Can you work these out from the model? Positions are in its coordinate system, mm. Give positions to 0.01 mm unless a question says otherwise; leave off trailing zeros. Order: outer loops, then holes, each group sorted by start corner. A loop starts at its lowest first (then second) coordinate and runs counter-clockwise, first axis right, second up.
Item 1: I want a section at D-D, the plane z = 2.1. Write out the boundary of the cut face in (x, y) (3 decimals).
Item 2: I want a section at C-C, the plane x = 40. Write out the boundary of the cut face in (y, z) (3 decimals).
Item 3: If we mould it in two halves opening along Y, with no side actions, what happens to faces 1 (the flat face through (25, 0, 2)), 2 (the flat face through (25, -47, 5)), 3 (the cylindrical face through (24.57, -85.48, 2.46))? For each: +Y half, -Y half, draft (parallel to the pull), parting line (faces both ways), or undercut.
Item 4: I want a section at A-A, the plane x = 25. Write out the boundary of the cut face in (y, z) (3 decimals), then the cut area to 3 significant figures.
Item 5: I want a section at B-B, the plane y = -9.5. Write out the boundary of the cut face in (x, z).
Item 6: If I drill on line 1 along Y through (x, z) = (10, 1.25) (3 decimals); line 2 along Y through (x, z) = (25, 3.5) (3 decimals); line 3 along Y through (x, z) = (39, 0.9), over which ranges is the centre line in solid material (lowest first)?
```python
from build123d import *

# Parameters (mm, degrees)
SKETCH1_W           = 50
SKETCH1_H           = 95
SKETCH1_R           = 2.5
SKETCH1_R_2         = 8
SKETCH1_R_3         = 2
BOSS_EXTRUDE1_DEPTH = 5
FILLET1_R           = 5


with BuildPart() as part:
    # Sketch1 → Boss-Extrude1 (new body)
    with BuildSketch(Plane.XY):
        with Locations((25, -47.5)):
            Rectangle(SKETCH1_W, SKETCH1_H)
        with Locations((10, -9.5)):
            Circle(SKETCH1_R, mode=Mode.SUBTRACT)
        with Locations((40, -9.5)):
            Circle(SKETCH1_R, mode=Mode.SUBTRACT)
        with Locations((25, -68.525)):
            Circle(SKETCH1_R_2, mode=Mode.SUBTRACT)
        with Locations((25, -53.525)):
            Circle(SKETCH1_R_3, mode=Mode.SUBTRACT)
        with Locations((40, -68.525)):
            Circle(SKETCH1_R_3, mode=Mode.SUBTRACT)
        with Locations((25, -83.525)):
            Circle(SKETCH1_R_3, mode=Mode.SUBTRACT)
        with Locations((10, -68.525)):
            Circle(SKETCH1_R_3, mode=Mode.SUBTRACT)
    extrude(amount=BOSS_EXTRUDE1_DEPTH)

    # Fillet1
    fillet1_edges = [part.edges().sort_by_distance(p)[0] for p in [
        (0, 0, 2.5),
        (50, 0, 2.5),
        (50, -95, 2.5),
        (0, -95, 2.5),
    ]]
    fillet(fillet1_edges, radius=FILLET1_R)


solid = part.part
```
Results list:
1. outline: (0, -90) arc R5 ccw to (5, -95) - (45, -95) arc R5 ccw to (50, -90) - (50, -5) arc R5 ccw to (45, 0) - (5, 0) arc R5 ccw to (0, -5) - close; hole circle Ø5 at (10, -9.5); hole circle Ø4 at (10, -68.525); hole circle Ø16 at (25, -68.525); hole circle Ø4 at (25, -83.525); hole circle Ø4 at (25, -53.525); hole circle Ø5 at (40, -9.5); hole circle Ø4 at (40, -68.525)
2. outline: (-95, 0) - (-70.525, 0) - (-70.525, 5) - (-95, 5) - close; (-66.525, 0) - (-12, 0) - (-12, 5) - (-66.525, 5) - close; (-7, 0) - (0, 0) - (0, 5) - (-7, 5) - close
3. face 1: +Y half
3. face 2: draft
3. face 3: undercut
4. outline: (-95, 0) - (-85.525, 0) - (-85.525, 5) - (-95, 5) - close; (-81.525, 0) - (-76.525, 0) - (-76.525, 5) - (-81.525, 5) - close; (-60.525, 0) - (-55.525, 0) - (-55.525, 5) - (-60.525, 5) - close; (-51.525, 0) - (0, 0) - (0, 5) - (-51.525, 5) - close
4. area: 355 mm2
5. outline: (0, 0) - (7.5, 0) - (7.5, 5) - (0, 5) - close; (12.5, 0) - (37.5, 0) - (37.5, 5) - (12.5, 5) - close; (42.5, 0) - (50, 0) - (50, 5) - (42.5, 5) - close
6. line 1: y = -95 to -70.525, -66.525 to -12, -7 to 0
6. line 2: y = -95 to -85.525, -81.525 to -76.525, -60.525 to -55.525, -51.525 to 0
6. line 3: y = -95 to -70.26, -66.79 to -11.79, -7.21 to 0
